Part model, mm, in its own coordinate system. A direction names the side the tool comes from. Give positions to 0.01 mm unless a question says otherwise; leave off trailing zeros. Write each loop counter-clockwise with the first axis right and the second up, starting at its lowest first coordinate (ties: lowest second). Pieces come first, ordered by that corner, then holes. Notation, with made-up numbers: M -3.5,82.25 L 39.5,82.25 A23 cw 39.5,118.25 Z; hole C 8,-16.75 d5. An arc over 180 degrees is marked long. Answer as CSV lines item,"result". Start each with the question number.
1) Slice it at B-B, the plane x = -13.5. Give the cut face in (y, z).
2) Wall check: line 1 along Z through (x, y) = (0.5, -10.75); line 2 along Z through (x, y) = (-15, -8.5). Give the ranges that are in metal, low to high. Write a range as from..to.
3) Tool access for faces 1 (the cylindrical face through (-40, -10, 0)), 2 (the flat face through (-2, -10, -38.5)), 3 (the flat face through (25, 0, -26)), 4 (the flat face through (26, -10, 26)), 5 (the flat face through (0, -11, -27.5)): list every direction of +Z, -Z, +X, -X, +Y, -Y with a clear straight run to the whole face (end or side of a thin tool).
4) Slice it at A-A, the plane z = 12.5. Give the cut face in (x, y), plus the area to 3 significant figures.
5) Pin check, flat tips, straight feed: pin 1 Ø3 at (x, z) = (-25, 27) entering from -Y; pin 2 Ø1.7 at (x, z) = (26.5, 25) entering from -Y; pin 3 Ø6 at (x, y) = (32, -11) entering from -Z. Stop position of each tip, or through.
6) Slice it at D-D, the plane z = 0. Give the cut face in (x, y).
7) Mould opens along X. For faces 6 (the flat face through (-31.81, -12.97, -23.37)), 7 (the flat face through (0, -7, 41)) say: pulls with the +X half, pulls with the -X half, needs draft (parallel to the pull), parting line crosses it, or undercut.
8) Slice it at C-C, the plane y = -8.75. Give the number of separate pieces and of enclosed holes in the cut face, plus the area to 3 significant figures.
```python
from build123d import *

# Parameters (mm, degrees)
SKETCH1_W           = 82
SKETCH1_H           = 82
SKETCH1_W_2         = 55
SKETCH1_H_2         = 55
BOSS_EXTRUDE1_DEPTH = 15
SKETCH2_R           = 10
CUT_EXTRUDE1_DEPTH  = 60.891568689
CUT_EXTRUDE2_START  = -30.5
SKETCH3_R           = 11
CUT_EXTRUDE2_DEPTH  = 8
CIRPATTERN3_COUNT   = 3
CIRPATTERN3_ANGLE   = 180
FILLET1_SIZE        = 11
CHAMFER1_SIZE       = 17
CUT_EXTRUDE3_START  = -7
CUT_EXTRUDE3_DEPTH  = 4
SKETCH5_R           = 2
CUT_EXTRUDE4_DEPTH  = 59.83876289
CIRPATTERN4_COUNT   = 4


with BuildPart() as part:
    # Sketch1 → Boss-Extrude1 (new body)
    with BuildSketch(Plane(origin=(0, 0, 0), x_dir=(1, 0, 0), z_dir=(0, 1, 0))):
        Rectangle(SKETCH1_W, SKETCH1_H)
        Rectangle(SKETCH1_W_2, SKETCH1_H_2, mode=Mode.SUBTRACT)
    extrude(amount=-BOSS_EXTRUDE1_DEPTH)

    # Sketch2 → Cut-Extrude1 (cut, through all)
    with BuildSketch(Plane(origin=(0, 0, 0), x_dir=(0, 0, -1), z_dir=(1, 0, 0))):
        Circle(SKETCH2_R)
    cut_extrude1 = extrude(amount=-CUT_EXTRUDE1_DEPTH, mode=Mode.SUBTRACT)

    # Sketch3 → Cut-Extrude2 (cut)
    with BuildSketch(Plane(origin=(0, 0, 0), x_dir=(0, 0, -1), z_dir=(1, 0, 0)).offset(CUT_EXTRUDE2_START)):
        Circle(SKETCH3_R)
    cut_extrude2 = extrude(amount=-CUT_EXTRUDE2_DEPTH, mode=Mode.SUBTRACT)

    # CirPattern3: Cut-Extrude1, Cut-Extrude2 ×3 about axis
    cirpattern3_axis = Axis((0, 0, 0), (0, -1, 0))
    add([cut_extrude1.rotate(cirpattern3_axis, i * CIRPATTERN3_ANGLE / (CIRPATTERN3_COUNT - 1)) for i in range(1, CIRPATTERN3_COUNT)], mode=Mode.SUBTRACT)
    add([cut_extrude2.rotate(cirpattern3_axis, i * CIRPATTERN3_ANGLE / (CIRPATTERN3_COUNT - 1)) for i in range(1, CIRPATTERN3_COUNT)], mode=Mode.SUBTRACT)

    # Fillet1
    # a fillet whose section is not a circle: 11 mm, written as the material it adds along each edge
    with BuildSketch(Plane(origin=(-27.5, 0, 27.5), x_dir=(0, 0, -1), z_dir=(0, -1, 0))) as fillet1_piece_1:
        with BuildLine():
            Bezier((FILLET1_SIZE, 0), (0, 0), (0, FILLET1_SIZE), weights=[1, 0.25, 1])
            Line((0, FILLET1_SIZE), (0, 0))
            Line((0, 0), (FILLET1_SIZE, 0))
        make_face()
    extrude(amount=15)
    with BuildSketch(Plane(origin=(-27.5, 0, -27.5), x_dir=(0, 0, 1), z_dir=(0, -1, 0)), Plane(origin=(27.5, 0, 27.5), x_dir=(0, 0, -1), z_dir=(0, -1, 0)), Plane(origin=(27.5, 0, -27.5), x_dir=(-1, 0, 0), z_dir=(0, -1, 0))) as fillet1_piece_2:
        with BuildLine():
            Bezier((FILLET1_SIZE, 0), (0, 0), (0, -FILLET1_SIZE), weights=[1, 0.25, 1])
            Line((0, -FILLET1_SIZE), (0, 0))
            Line((0, 0), (FILLET1_SIZE, 0))
        make_face()
    extrude(amount=15)

    # Chamfer1
    chamfer1_edges = [part.edges().sort_by_distance(p)[0] for p in [
        (41, -7.5, 41),
        (-41, -7.5, 41),
        (-41, -7.5, -41),
        (41, -7.5, -41),
    ]]
    chamfer(chamfer1_edges, length=CHAMFER1_SIZE)

    # Sketch4 → Cut-Extrude3 (cut, symmetric)
    with BuildSketch(Plane(origin=(32.5, 0, -32.5), x_dir=(-0.7071067811865488, 0, -0.7071067811865464), z_dir=(0.7071067811865464, 0, -0.7071067811865488)).offset(CUT_EXTRUDE3_START)):
        Polygon((-2, -10), (2, -10), (2, -11), (4, -11), (8, -15), (-8, -15), (-4, -11), (-2, -11), align=None)
    cut_extrude3 = extrude(amount=CUT_EXTRUDE3_DEPTH, both=True, mode=Mode.SUBTRACT)

    # Sketch5 → Cut-Extrude4 (cut, through all)
    with BuildSketch(Plane.XZ.offset(10)):
        with Locations(Location((27.550252532, -27.550252532, 0), (0, 0, 225))):
            Circle(SKETCH5_R)
    cut_extrude4 = extrude(amount=-CUT_EXTRUDE4_DEPTH, mode=Mode.SUBTRACT)

    # CirPattern4: Cut-Extrude3, Cut-Extrude4 ×4 about axis
    cirpattern4_axis = Axis((0, 0, 0), (0, 1, 0))
    add([cut_extrude3.rotate(cirpattern4_axis, i * 360 / CIRPATTERN4_COUNT) for i in range(1, CIRPATTERN4_COUNT)], mode=Mode.SUBTRACT)
    add([cut_extrude4.rotate(cirpattern4_axis, i * 360 / CIRPATTERN4_COUNT) for i in range(1, CIRPATTERN4_COUNT)], mode=Mode.SUBTRACT)


solid = part.part
```
Found:
1,outline,"M -15,-41 L 0,-41 L 0,-27.5 L -15,-27.5 Z; M -15,27.5 L 0,27.5 L 0,41 L -15,41 Z"
2,line 1,"-41..-38.5, -30.5..-27.5, 27.5..41"
2,line 2,"-41..-27.5, 27.5..41"
3,face 1,"+X, -X, +Y"
3,face 2,"+Y"
3,face 3,"+Z, -Z, +X, -X, +Y"
3,face 4,"-Y"
3,face 5,"+Y, -Y"
4,outline,"M -41,-15 L -27.5,-15 L -27.5,0 L -41,0 Z; M 27.5,-15 L 41,-15 L 41,0 L 27.5,0 Z"
4,area,"405 mm²"
5,pin 1,"y = -11"
5,pin 2,"y = -10"
5,pin 3,"z = -36"
6,outline,"M -41,-15 L -27.5,-15 L -27.5,-10 L -30.5,-10 L -30.5,-11 L -38.5,-11 L -38.5,-10 L -41,-10 Z; M 27.5,-15 L 41,-15 L 41,-10 L 38.5,-10 L 38.5,-11 L 30.5,-11 L 30.5,-10 L 27.5,-10 Z"
7,face 6,"undercut"
7,face 7,"needs draft"
8,separate pieces,"3"
8,enclosed holes,"4"
8,area,"2,760 mm²"
